For this review, use the dimensioned drawing (mm, ordinates from the lowest corner) and the shaded views. A direction names the side the tool comes from. Coordinates: 2 decimals unless noted, no trailing zeros. Loops run counter-clockwise (first coordinate to the right, second up) from the corner with the lowest first, then second, coordinate; pieces in that order, holes last. Notation, with made-up numbers: (28.5, -5.75) -> (50.5, -5.75) arc R17 ccw to (50.5, 7.25) -> close; hole circle Ø4 at (42.5, 14). An arc over 180 degrees is marked (long way). Use one line per item in the form item = value. Start each with the question number.
1. Consider section C-C (y = 9.25). State the section outline as (x, z) points.
2. The part is to be moulded in two halves that separate along X. For the marked faces 3, 4 and 5, say which applies: released by +X, released by -X, zero draft, split by the parting line, or undercut.
3. Consider section A-A (x = 3.46). State the section outline as (y, z) points.
4. Machinability: for the marked faces 1 and 2, which of the approach directions +Z, -Z, +X, -X, +Y, -Y give a long, thin tool a straight path to every point of the face, cutting with its end or side? Answer none if there is none.
5. For pin 1 (0.5 mm diameter, centred on y = 11.5, z = 2.5, fed in from +X); pin 2 (2 mm diameter, centred on y = 3.5, z = 3.5, fed in from +X); pin 3 (1.1 mm diameter, centred on y = 11.5, z = 2.5, fed in from -X), all flat-tipped, find the tip position at first contact; note any pin that passes through.
6. Consider section D-D (x = 5.75). State the section outline as (y, z) points.
7. Wall thickness on line 1 (Y direction, x = 5.75, z = 1); line 2 (Y direction, x = 3, z = 3.25); line 3 (Z direction, x = 3.5, y = 9.25): over which ranges is each line inside the solid? List them lowest first. Write a range as from..to.
8. Consider section B-B (z = 3.46). State the section outline as (x, y) points, then the cut area to 3 significant figures.
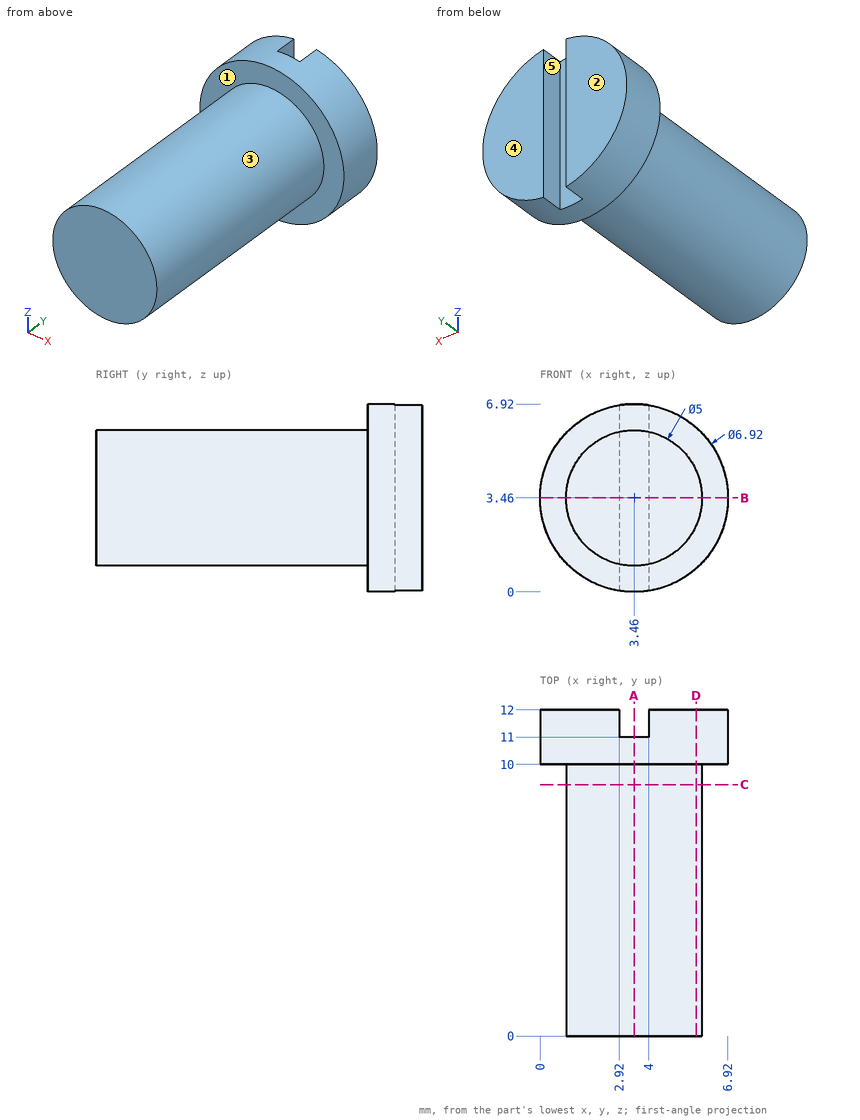
Geometry check:
q1.outline = circle Ø5 at (3.46, 3.46)
q2.face_3 = split by the parting line
q2.face_4 = zero draft
q2.face_5 = undercut
q3.outline = (0, 0.96) -> (10, 0.96) -> (10, 0) -> (11, 0) -> (11, 6.92) -> (10, 6.92) -> (10, 5.96) -> (0, 5.96) -> close
q4.face_1 = -Y
q4.face_2 = +Z, -Z, +X, -X, +Y
q5.pin_1 = 6.85
q5.pin_2 = 5.96
q5.pin_3 = 0.02
q6.outline = (0, 2.46) -> (10, 2.46) -> (10, 0.87) -> (12, 0.87) -> (12, 6.05) -> (10, 6.05) -> (10, 4.46) -> (0, 4.46) -> close
q7.line_1 = 10..12
q7.line_2 = 0..11
q7.line_3 = 0.96..5.96
q8.outline = (0, 10) -> (0.96, 10) -> (0.96, 0) -> (5.96, 0) -> (5.96, 10) -> (6.92, 10) -> (6.92, 12) -> (4, 12) -> (4, 11) -> (2.92, 11) -> (2.92, 12) -> (0, 12) -> close
q8.area = 62.8 mm²
